from build123d import *

# Parameters (mm, degrees)
F0_R     = 12.7
F1_DEPTH = 381
F3_DEPTH = 15.875
F4_R     = 6.35
F5_DEPTH = 12.7


with BuildPart() as f1:
    # F0 (on Top) → F1 (new body)
    with BuildSketch(Plane.XY):
        Circle(F0_R)
    extrude(amount=F1_DEPTH)

    # F2 (on face) → F3 (join)
    with BuildSketch(Plane.XY.offset(381)):
        with BuildLine():
            ThreePointArc((-4.7625, -6.35), (0, -7.9375), (4.7625, -6.35))
            Line((4.7625, -6.35), (-4.7625, -6.35))
        make_face()
        Polygon((4.7625, 0), (4.7625, 6.35), (-4.7625, 6.35), (-4.7625, 0), (-4.7625, -6.35), (4.7625, -6.35), align=None)
        with BuildLine():
            Line((-4.7625, 6.35), (4.7625, 6.35))
            ThreePointArc((4.7625, 6.35), (0, 7.9375), (-4.7625, 6.35))
        make_face()
    extrude(amount=F3_DEPTH)

    # F4 (on face) → F5 (join)
    with BuildSketch(Plane(origin=(0, 0, 0), x_dir=(1, 0, 0), z_dir=(0, 0, -1))):
        Circle(F4_R)
    extrude(amount=F5_DEPTH)


solid = f1.part
CAD build for the part. Positions are in the model's coordinates, mm. A direction names the side the tool comes from. Round coordinates to 2 decimals unless told otherwise and drop trailing zeros. Loops run counter-clockwise (first coordinate to the right, second up) from the corner with the lowest first, then second, coordinate; pieces in that order, holes last.
(1) Drop flat-ended pins along their axis: pin 1 (10 mm diameter, centred on y = 3, z = 392.5, fed in from -X); pin 2 (2 mm diameter, centred on y = -1.5, z = 88.5, fed in from -X); pin 3 (1.5 mm diameter, centred on x = 4, z = 266, fed in from -Y). Give the stop position or say it passes through.
(2) Cut at B-B (x = 1). Give the cut face in (y, z) (3 decimals).
(3) Wall check: line 1 along Z through (x, y) = (8, 0.5); line 2 along Y through (x, z) = (-1.25, 69); line 3 along X through (y, z) = (-0.75, 224). Give the ranges that are in metal, low to high.
(4) Two-plate mould, pull along Y, no slides. Class faces 6 (the cylindrical face through (-0.072, -7.937, 388.826)), 7 (the flat face through (4.762, 0, 389)), 8 (the cylindrical face through (0.072, 7.937, 388.826)): +Y half, -Y half, draft (parallel to the pull), parting line (faces both ways), or undercut.
(5) Which spindle directions (+Z, -Z, +X, -X, +Y, -Y) get a long thin tool onto all of the face, cutting with end or side? Do faces 1 (the flat face through (0, 0, -12.7)), 2 (the cylindrical face through (-2.75, -12.4, 187.83)), 3 (the cylindrical face through (-1.38, 6.2, -6.26)), 4 (the flat face through (5, 0, 381)), 5 (the flat face through (-4.762, 0, 389)). Say none if no direction does.
(6) Cut at C-C (z = 240). Give the cut face in (x, y), plus the area to 3 significant figures.
Findings below:
1. pin 1: stops at x = -4.76
1. pin 2: stops at x = -12.69
1. pin 3: stops at y = -12.28
2. outline: (-12.661, 0) - (-6.271, 0) - (-6.271, -12.7) - (6.271, -12.7) - (6.271, 0) - (12.661, 0) - (12.661, 381) - (7.874, 381) - (7.874, 396.875) - (-7.874, 396.875) - (-7.874, 381) - (-12.661, 381) - close
3. line 1: z = 0 to 381
3. line 2: y = -12.64 to 12.64
3. line 3: x = -12.68 to 12.68
4. face 6: -Y half
4. face 7: draft
4. face 8: +Y half
5. face 1: -Z, +X, -X, +Y, -Y
5. face 2: +Z, -Z
5. face 3: -Z
5. face 4: +Z
5. face 5: +Z, -X, +Y, -Y
6. outline: circle Ø25.4 at (0, 0)
6. area: 507 mm2
